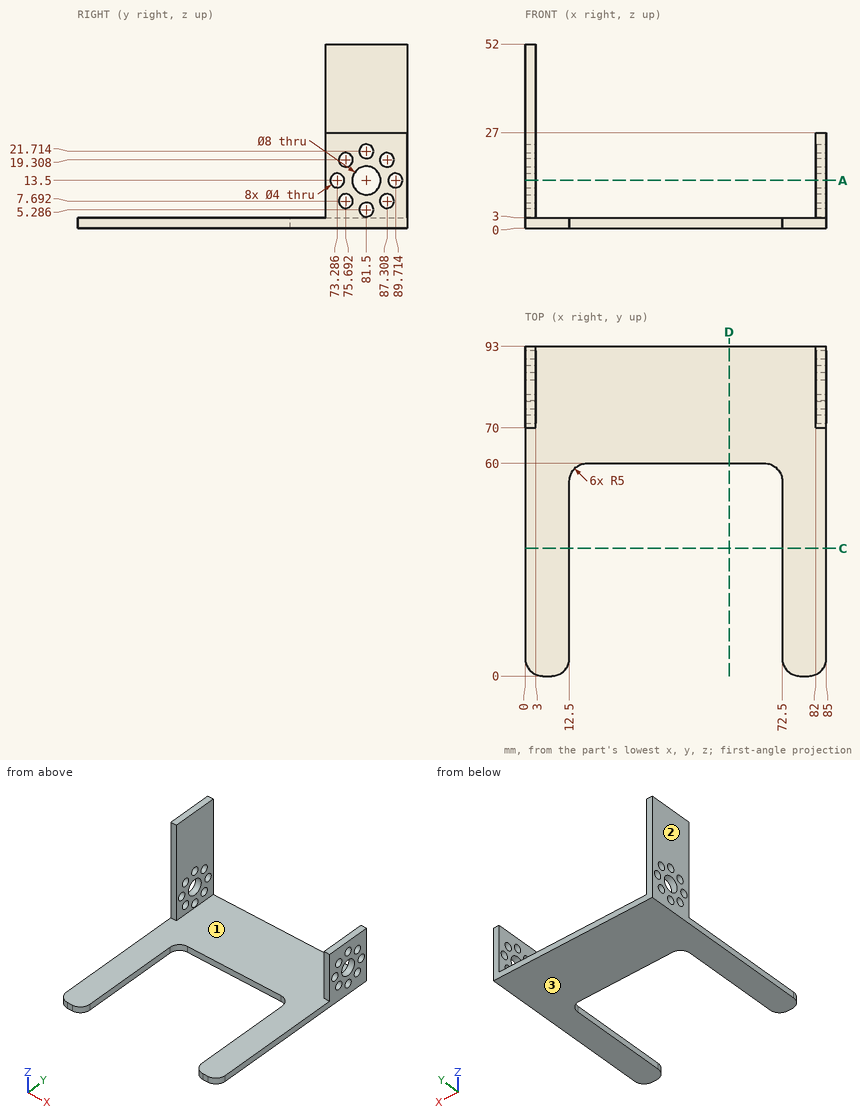
Job drawing, mm, ordinate dimensions from the low corner. One solid piece. Round coordinates to 2 decimals unless told otherwise and drop trailing zeros. Loops run counter-clockwise (first coordinate to the right, second up) from the corner with the lowest first, then second, coordinate; pieces in that order, holes last.
(1) Cut at C-C (y = 36). Give the cut face in (x, z), plus the area to 3 significant figures.
(2) Cut at D-D (x = 57.5). Give the cut face in (y, z), plus the area to 3 significant figures.
(3) Two-plate mould, pull along X, no slides. Class the marked faces 1, 2 and 3: +X half, -X half, draft (parallel to the pull), parting line (faces both ways), or undercut.
(4) Drop flat-ended pins along their axis: pin 1 (8 mm diameter, centred on x = 18, y = 20, fed in from +Z); pin 2 (6.5 mm diameter, centred on y = 81.5, z = 5.29, fed in from +X); pin 3 (3.5 mm diameter, centred on x = 37, z = 1, fed in from -Y). Give the stop position or say it passes through.
(5) Wall check: line 1 along X through (y, z) = (30, 2.5); line 2 along Z through (x, y) = (83, 81); line 3 along X through (y, z) = (81, 44). Give the ranges that are in metal, low to high.
(6) Cut at A-A (z = 13.5). State how many separate pieces and enclosed holes the cut face has, plus the area to 3 significant figures.
Findings below:
1. outline: (0, 0) - (12.5, 0) - (12.5, 3) - (0, 3) - close; (72.5, 0) - (85, 0) - (85, 3) - (72.5, 3) - close
1. area: 75.0 mm2
2. outline: (60, 0) - (93, 0) - (93, 3) - (60, 3) - close
2. area: 99.0 mm2
3. face 1: undercut
3. face 2: -X half
3. face 3: draft
4. pin 1: passes through
4. pin 2: stops at x = 85
4. pin 3: stops at y = 60
5. line 1: x = 0 to 12.5, 72.5 to 85
5. line 2: z = 0 to 3.35, 7.22 to 9.53, 17.47 to 19.78, 23.65 to 27
5. line 3: x = 0 to 3
6. separate pieces: 8
6. enclosed holes: 0
6. area: 42.0 mm2
